```python
from build123d import *

# Parameters (mm, degrees)
SKETCH1_R           = 3.4
BOSS_EXTRUDE1_DEPTH = 5
SKETCH3_W           = 6
SKETCH3_H           = 1.5
BOSS_EXTRUDE2_DEPTH = 5
FILLET2_R           = 1.5
FILLET3_R           = 1


with BuildPart() as part:
    # Sketch1 → Boss-Extrude1 (new body)
    with BuildSketch(Plane(origin=(0, 0, 0), x_dir=(0, 0, -1), z_dir=(1, 0, 0))):
        Polygon((2.5, 0), (8.5, 0), (8.5, 3.5), (11, 3.5), (11, 13.5), (8.5, 13.5), (8.5, 17), (2.5, 17), (2.5, 13.5), (0, 13.5), (0, 3.5), (2.5, 3.5), align=None)
        with Locations((5.5, 8.5)):
            Circle(SKETCH1_R, mode=Mode.SUBTRACT)
    extrude(amount=BOSS_EXTRUDE1_DEPTH)

    # Sketch3 → Boss-Extrude2 (add)
    with BuildSketch(Plane.ZY):
        with Locations((-5.5, 16.25)):
            Rectangle(SKETCH3_W, SKETCH3_H)
        with Locations((-5.5, 0.75)):
            Rectangle(SKETCH3_W, SKETCH3_H)
    extrude(amount=BOSS_EXTRUDE2_DEPTH)

    # Fillet2
    fillet2_edges = [part.edges().sort_by_distance(p)[0] for p in [
        (2.5, 13.5, -8.5),
        (2.5, 13.5, -2.5),
        (2.5, 3.5, -2.5),
        (2.5, 3.5, -8.5),
    ]]
    fillet(fillet2_edges, radius=FILLET2_R)

    # Fillet3
    fillet3_edges = [part.edges().sort_by_distance(p)[0] for p in [
        (2.5, 3.5, -11),
        (2.5, 3.5, 0),
        (2.5, 13.5, 0),
        (2.5, 13.5, -11),
    ]]
    fillet(fillet3_edges, radius=FILLET3_R - 0.0001)  # a hair under: the kernel refuses the full size


solid = part.part
```
Could you check a few things on this model? Use its own coordinates, in mm. A direction names the side the tool comes from. Coordinates: 2 decimals unless noted, no trailing zeros. Loops run counter-clockwise (first coordinate to the right, second up) from the corner with the lowest first, then second, coordinate; pieces in that order, holes last.
1) Will these pins go through, and if not, where does the flat tip stop? pin 1 Ø5.5 at (y, z) = (5, -6.5) entering from -X; pin 2 Ø2 at (x, z) = (2.5, -5) entering from -Y; pin 3 Ø2 at (x, y) = (1, 16) entering from -Z; pin 4 Ø1 at (x, y) = (1.5, 0.5) entering from +Z.
Reported:
pin 1: stops at x = 0
pin 2: stops at y = 0
pin 3: stops at z = -8.5
pin 4: stops at z = -2.5
2) Thinking about a two-plate mould opening in Y: for faces 1 (the face through (2.54, 13.95, -8.93)), 2 (the face through (0, 16, -2.5)), 3 (the face through (-2, 1.5, -6)), which applies, released by +Y, released by -Y, zero draft, split by the parting line, or undercut?
Reported:
face 1: released by +Y
face 2: zero draft
face 3: undercut
3) Please list where these lines run through material, in increasing order: line 1 along Y through (x, z) = (1.7, -5.5); line 2 along X through (y, z) = (8.25, -9.25); line 3 along Y through (x, z) = (-3, -8.25).
Reported:
line 1: y = 0 to 5.1, 11.9 to 17
line 2: x = 0 to 5
line 3: y = 0 to 1.5, 15.5 to 17
4) Imagine slicing it at C-C (z = -5.5). List the corners of the cut face in (x, y) for me, and give its area (3 significant figures).
Reported:
outline: (-5, 0) - (5, 0) - (5, 5.1) - (0, 5.1) - (0, 1.5) - (-5, 1.5) - close; (-5, 15.5) - (0, 15.5) - (0, 11.9) - (5, 11.9) - (5, 17) - (-5, 17) - close
area: 66.0 mm2
5) Which directions (+Z, -Z, +X, -X, +Y, -Y) give clear straight access to the entire face, cutting with the end or side of a thin tool? Please do faces 4 (the face through (2.54, 13.95, -2.07)), 5 (the face through (0, 16, -8.5)), 6 (the face through (-5, 1, -6)), 7 (the face through (0, 1, -8.5)), 8 (the face through (0, 12, -7)).
Reported:
face 4: +Z, +X, -X, +Y
face 5: -Z, +X, -X, +Y
face 6: +Z, -Z, -X, +Y, -Y
face 7: -Z, +X, -X, -Y
face 8: +Z, -Z, -X
6) Imagine slicing it at A-A (y = 8.5). List the corners of the cut face in (x, z) for me, and give its area (3 significant figures).
Reported:
outline: (0, -11) - (5, -11) - (5, -8.9) - (0, -8.9) - close; (0, -2.1) - (5, -2.1) - (5, 0) - (0, 0) - close
area: 21.0 mm2
7) Imagine slicing it at B-B (x = -0.5). List the corners of the cut face in (y, z) for me, and give its area (3 significant figures).
Reported:
outline: (0, -8.5) - (1.5, -8.5) - (1.5, -2.5) - (0, -2.5) - close; (15.5, -8.5) - (17, -8.5) - (17, -2.5) - (15.5, -2.5) - close
area: 18.0 mm2
